Could you check a few things on this model? Use its own coordinates, in mm. A direction names the side the tool comes from. Give positions to 0.01 mm unless a question says otherwise; leave off trailing zeros. Order: outer loops, then holes, each group sorted by start corner. A loop starts at its lowest first (then second) coordinate and runs counter-clockwise, first axis right, second up. Notation, with made-up numbers: (70.25, 25) -> (106.25, 25) arc R15 cw to (106.25, 29) -> close; hole circle Ø9 at (62.5, 23). An arc over 180 degrees is marked (long way). Answer as CSV lines item,"result". Start each with the question number.
(1) I want a section at B-B (y = 202). Please give me the cut outline in (x, z), plus the area to 3 significant figures.
(2) We'd pull the mould along X, two halves only. Please class faces 1 (the face through (-74, 255, 19.5)), 2 (the face through (83.33, 263.645, 6.844)), 3 (the face through (0.2, 0.7, 10.5)), 4 (the face through (-100.776, 165.584, 17.937)): released by +X, released by -X, zero draft, split by the parting line, or undercut.
(3) I want a section at C-C (z = 4.5). Give the number of separate pieces and of enclosed holes in the cut face, plus the area to 3 significant figures.
(4) On a 3-axis mill with a long thin cutter (end or side, diameter ignored), from which of +Z, -Z, +X, -X, +Y, -Y can I reach the whole of each face in a straight line? I mean faces 5 (the face through (42, 43, 9.5)), 6 (the face through (-1, 280.197, 11)), 7 (the face through (44, 13, 10)). Say none if no direction works.
(5) I want a section at A-A (x = -24). Please give me the cut outline in (y, z).
(6) Will these pins go through, and if not, where does the flat tip stop? pin 1 Ø3.5 at (y, z) = (5.5, 5.5) entering from -X; pin 2 Ø8 at (x, z) = (23, 18.5) entering from -Y; pin 3 Ø7 at (y, z) = (40.5, 6) entering from +X.
(7) I need wall thicknesses on L1, parallel to X at y = 53, z = 12.5; L2, parallel to X at y = 194.5, z = 8.25; L3, parallel to Y at x = 45.5, z = 15. Which ranges of each line are inside material? Lowest first, please.
```python
from build123d import *

# Parameters (mm, degrees)
RESSALTO_EXTRUS_O1_DEPTH = 22.5
CHANFRO1_SIZE            = 9
CORTE_EXTRUS_O1_REACH    = 24.5
ESBO_O3_W                = 1139.230904301
ESBO_O3_H                = 709.798033895
CORTE_EXTRUS_O5_DEPTH    = 3
CORTE_EXTRUS_O6_REACH    = 21.5
ESBO_O5_W                = 77
ESBO_O5_H                = 10
ESBO_O7_R                = 2.1
ESBO_O7_R_2              = 2.15
CORTE_EXTRUS_O7_DEPTH    = 23.5
CORTE_EXTRUS_O8_DEPTH    = 10
ESBO_O9_W                = 92.788829696
ESBO_O9_H                = 85.062360753
CORTE_EXTRUS_O9_DEPTH    = 23.5
CORTE_EXTRUS_O10_REACH   = 21.5
CORTE_EXTRUS_O11_DEPTH   = 7
ESBO_O12_R               = 10.5
CORTE_EXTRUS_O12_DEPTH   = 7
CORTE_EXTRUS_O13_DEPTH   = 10


with BuildPart() as part:
    # Esboço1 → Ressalto-extrusão1 (new body, symmetric)
    with BuildSketch(Plane.XY):
        with BuildLine():
            Line((-56.387503511, 290.197344596), (56.387503511, 290.197344596))
            ThreePointArc((56.387503511, 290.197344596), (60.613686129, 289.260422466), (64.047947942, 286.625220692))
            Line((64.047947942, 286.625220692), (103.160444431, 240.012762487))
            ThreePointArc((103.160444431, 240.012762487), (104.896926208, 237.005087823), (105.5, 233.58488639))
            Line((105.5, 233.58488639), (105.5, 167.188670131))
            ThreePointArc((105.5, 167.188670131), (104.953136861, 164.08725515), (103.378507208, 161.359916588))
            Line((103.378507208, 161.359916588), (62.621492792, 112.787598236))
            ThreePointArc((62.621492792, 112.787598236), (61.046863139, 110.060259674), (60.5, 106.958844693))
            Line((60.5, 106.958844693), (60.5, 10.605625498))
            ThreePointArc((60.5, 10.605625498), (59.56307787, 6.379442881), (56.927876097, 2.945181067))
            Line((56.927876097, 2.945181067), (55.249552272, 1.536900164))
            ThreePointArc((55.249552272, 1.536900164), (52.241877608, -0.199581612), (48.821676175, -0.802655404))
            Line((48.821676175, -0.802655404), (-48.821676175, -0.802655404))
            ThreePointArc((-48.821676175, -0.802655404), (-52.241877608, -0.199581612), (-55.249552272, 1.536900164))
            Line((-55.249552272, 1.536900164), (-56.927876097, 2.945181067))
            ThreePointArc((-56.927876097, 2.945181067), (-59.56307787, 6.379442881), (-60.5, 10.605625498))
            Line((-60.5, 10.605625498), (-60.5, 106.958844693))
            ThreePointArc((-60.5, 106.958844693), (-61.046863139, 110.060259674), (-62.621492792, 112.787598236))
            Line((-62.621492792, 112.787598236), (-103.378507208, 161.359916588))
            ThreePointArc((-103.378507208, 161.359916588), (-104.953136861, 164.08725515), (-105.5, 167.188670131))
            Line((-105.5, 167.188670131), (-105.5, 233.58488639))
            ThreePointArc((-105.5, 233.58488639), (-104.896926208, 237.005087823), (-103.160444431, 240.012762487))
            Line((-103.160444431, 240.012762487), (-64.047947942, 286.625220692))
            ThreePointArc((-64.047947942, 286.625220692), (-60.613686129, 289.260422466), (-56.387503511, 290.197344596))
        make_face()
        Polygon((-48.869071975, 270.197344596), (48.869071975, 270.197344596), (83.5, 228.925811707), (83.5, 171.895558399), (38.5, 118.266646732), (38.5, 19.197344596), (-38.5, 19.197344596), (-38.5, 118.266646732), (-83.5, 171.895558399), (-83.5, 228.925811707), align=None, mode=Mode.SUBTRACT)
    extrude(amount=RESSALTO_EXTRUS_O1_DEPTH, both=True)

    # Chanfro1
    chanfro1_edges = [part.edges().sort_by_distance(p)[0] for p in [
        (83.604196187, 263.318991589, 22.5),
        (60.613686129, 289.260422466, 22.5),
        (0, 290.197344596, 22.5),
        (-60.613686129, 289.260422466, 22.5),
        (-83.604196187, 263.318991589, 22.5),
        (-104.896926208, 237.005087823, 22.5),
        (-105.5, 200.38677826, 22.5),
        (-104.953136861, 164.08725515, 22.5),
        (-83, 137.073757412, 22.5),
        (-61.046863139, 110.060259674, 22.5),
        (-60.5, 58.782235095, 22.5),
        (-59.56307787, 6.379442881, 22.5),
        (-56.088714184, 2.241040616, 22.5),
        (-52.241877608, -0.199581612, 22.5),
        (0, -0.802655404, 22.5),
        (52.241877608, -0.199581612, 22.5),
        (56.088714184, 2.241040616, 22.5),
        (59.56307787, 6.379442881, 22.5),
        (60.5, 58.782235095, 22.5),
        (61.046863139, 110.060259674, 22.5),
        (83, 137.073757412, 22.5),
        (104.953136861, 164.08725515, 22.5),
        (105.5, 200.38677826, 22.5),
        (104.896926208, 237.005087823, 22.5),
    ]]
    chamfer(chanfro1_edges, length=CHANFRO1_SIZE)

    # Esboço3 → Corte-extrusão1 (cut, up to next)
    with BuildSketch(Plane.XY, mode=Mode.PRIVATE) as corte_extrus_o1_sk1:
        with Locations((-153.157436203, 152.53565808)):
            Rectangle(ESBO_O3_W, ESBO_O3_H)
    corte_extrus_o1_tool1 = extrude(corte_extrus_o1_sk1.sketch, amount=-CORTE_EXTRUS_O1_REACH, mode=Mode.PRIVATE) & part.part
    add(corte_extrus_o1_tool1.solids().sort_by_distance((-153.157436, 152.535658, 0))[0], mode=Mode.SUBTRACT)

    # Esboço4 → Corte-extrusão5 (cut)
    with BuildSketch(Plane.XY.offset(22.5)):
        Polygon((56.387503511, 280.197344596), (-56.387503511, 280.197344596), (-95.5, 233.58488639), (-95.5, 167.527915588), (-50.5, 113.899003921), (-50.5, 10.605625498), (-48.821676175, 9.197344596), (48.821676175, 9.197344596), (50.5, 10.605625498), (50.5, 113.899003921), (95.5, 167.527915588), (95.5, 233.58488639), align=None)
        Polygon((38.5, 19.197344596), (-38.5, 19.197344596), (-38.5, 121.489121124), (-83.5, 175.11803279), (-83.5, 228.925811707), (-48.869071975, 270.197344596), (48.869071975, 270.197344596), (83.5, 228.925811707), (83.5, 175.11803279), (38.5, 121.489121124), align=None, mode=Mode.SUBTRACT)
    extrude(amount=-CORTE_EXTRUS_O5_DEPTH, mode=Mode.SUBTRACT)

    # Esboço5 → Corte-extrusão6 (cut, up to next)
    with BuildSketch(Plane.XY.offset(19.5), mode=Mode.PRIVATE) as corte_extrus_o6_sk1:
        Polygon((-95.5, 233.58488639), (-83.5, 228.925811707), (-83.5, 171.895558399), (-95.5, 167.527915588), align=None)
    corte_extrus_o6_tool1 = extrude(corte_extrus_o6_sk1.sketch, amount=-CORTE_EXTRUS_O6_REACH, mode=Mode.PRIVATE) & part.part
    add(corte_extrus_o6_tool1.solids().sort_by_distance((-89.646672, 200.485324, 19.5))[0], mode=Mode.SUBTRACT)
    # Esboço5 → Corte-extrusão6 (cut, up to next)
    with BuildSketch(Plane.XY.offset(19.5), mode=Mode.PRIVATE) as corte_extrus_o6_sk2:
        Polygon((-48.869071975, 270.197344596), (-56.387503511, 280.197344596), (56.387503511, 280.197344596), (48.869071975, 270.197344596), align=None)
    corte_extrus_o6_tool2 = extrude(corte_extrus_o6_sk2.sketch, amount=-CORTE_EXTRUS_O6_REACH, mode=Mode.PRIVATE) & part.part
    add(corte_extrus_o6_tool2.solids().sort_by_distance((0, 275.316394, 19.5))[0], mode=Mode.SUBTRACT)
    # Esboço5 → Corte-extrusão6 (cut, up to next)
    with BuildSketch(Plane.XY.offset(19.5), mode=Mode.PRIVATE) as corte_extrus_o6_sk3:
        with Locations((0, 14.197344596)):
            Rectangle(ESBO_O5_W, ESBO_O5_H)
    corte_extrus_o6_tool3 = extrude(corte_extrus_o6_sk3.sketch, amount=-CORTE_EXTRUS_O6_REACH, mode=Mode.PRIVATE) & part.part
    add(corte_extrus_o6_tool3.solids().sort_by_distance((0, 14.197345, 19.5))[0], mode=Mode.SUBTRACT)
    # Esboço5 → Corte-extrusão6 (cut, up to next)
    with BuildSketch(Plane.XY.offset(19.5), mode=Mode.PRIVATE) as corte_extrus_o6_sk4:
        Polygon((83.5, 171.895558399), (95.5, 167.527915588), (95.5, 233.58488639), (83.5, 228.925811707), align=None)
    corte_extrus_o6_tool4 = extrude(corte_extrus_o6_sk4.sketch, amount=-CORTE_EXTRUS_O6_REACH, mode=Mode.PRIVATE) & part.part
    add(corte_extrus_o6_tool4.solids().sort_by_distance((89.646672, 200.485324, 19.5))[0], mode=Mode.SUBTRACT)

    # Esboço7 → Corte-extrusão7 (cut, through all)
    with BuildSketch(Plane.XY.offset(22.5)):
        with Locations((-45.5, 14.923339275)):
            Circle(ESBO_O7_R)
        with Locations((-43.5, 44.856598369)):
            Circle(ESBO_O7_R_2)
        with Locations((-71.975269931, 253.84194883)):
            Circle(ESBO_O7_R)
        with Locations((-59.836146954, 265.197344596)):
            Circle(ESBO_O7_R_2)
        with Locations((59.836146954, 265.197344596)):
            Circle(ESBO_O7_R_2)
        with Locations((71.975269931, 253.84194883)):
            Circle(ESBO_O7_R)
        with Locations((43.5, 44.856598369)):
            Circle(ESBO_O7_R_2)
        with Locations((45.5, 14.923339275)):
            Circle(ESBO_O7_R)
        with Locations((-67.431100943, 144.966771084)):
            Circle(ESBO_O7_R_2)
        with Locations((67.431100943, 144.966771084)):
            Circle(ESBO_O7_R_2)
    extrude(amount=-CORTE_EXTRUS_O7_DEPTH, mode=Mode.SUBTRACT)

    # Esboço8 → Corte-extrusão8 (cut)
    with BuildSketch(Plane(origin=(0, 0, 0), x_dir=(-1, 0, 0), z_dir=(0, 0, -1))):
        Polygon((-73.397020968, 257.748177701), (-76.069038884, 254.56379075), (-74.647287847, 250.657561879), (-70.553518893, 249.93571996), (-67.881500977, 253.120106911), (-69.303252014, 257.026335782), align=None)
        Polygon((-45.5, 19.080261213), (-49.1, 17.001800244), (-49.1, 12.844878306), (-45.5, 10.766417337), (-41.9, 12.844878306), (-41.9, 17.001800244), align=None)
        Polygon((41.9, 17.001800244), (45.5, 19.080261213), (49.1, 17.001800244), (49.1, 12.844878306), (45.5, 10.766417337), (41.9, 12.844878306), align=None)
        Polygon((76.069038884, 254.56379075), (73.397020968, 257.748177701), (69.303252014, 257.026335782), (67.881500977, 253.120106911), (70.553518893, 249.93571996), (74.647287847, 250.657561879), align=None)
        Polygon((67.580931876, 147.478918378), (71.560985025, 146.777127623), (72.943242978, 142.97940511), (70.345447782, 139.883473352), (66.365394632, 140.585264107), (64.98313668, 144.38298662), align=None)
    extrude(amount=-CORTE_EXTRUS_O8_DEPTH, mode=Mode.SUBTRACT)

    # Esboço9 → Corte-extrusão9 (cut, through all)
    with BuildSketch(Plane.XY.offset(22.5)):
        with Locations((-70.062226852, 117.896927121)):
            Rectangle(ESBO_O9_W, ESBO_O9_H)
    extrude(amount=-CORTE_EXTRUS_O9_DEPTH, mode=Mode.SUBTRACT)

    # Esboço10 → Corte-extrusão10 (cut, up to next)
    with BuildSketch(Plane.XY.offset(19.5), mode=Mode.PRIVATE) as corte_extrus_o10_sk1:
        Polygon((-95.5, 167.527915588), (-83.5, 171.895558399), (-73.877666178, 160.428107498), (-89.54255365, 160.428107498), align=None)
    corte_extrus_o10_tool1 = extrude(corte_extrus_o10_sk1.sketch, amount=-CORTE_EXTRUS_O10_REACH, mode=Mode.PRIVATE) & part.part
    add(corte_extrus_o10_tool1.solids().sort_by_distance((-85.062746, 165.15554, 19.5))[0], mode=Mode.SUBTRACT)
    # Esboço10 → Corte-extrusão10 (cut, up to next)
    with BuildSketch(Plane.XY.offset(19.5), mode=Mode.PRIVATE) as corte_extrus_o10_sk2:
        Polygon((89.54255365, 160.428107498), (95.5, 167.527915588), (83.5, 171.895558399), (73.877666178, 160.428107498), align=None)
    corte_extrus_o10_tool2 = extrude(corte_extrus_o10_sk2.sketch, amount=-CORTE_EXTRUS_O10_REACH, mode=Mode.PRIVATE) & part.part
    add(corte_extrus_o10_tool2.solids().sort_by_distance((85.062746, 165.15554, 19.5))[0], mode=Mode.SUBTRACT)

    # Esboço11 → Corte-extrusão11 (cut)
    with BuildSketch(Plane(origin=(0, 9.197344596, 0), x_dir=(1, 0, 0), z_dir=(0, 1, 0))):
        Polygon((0, -15.703927322), (13.6, -7.851963661), (13.6, 7.851963661), (0, 15.703927322), (-13.6, 7.851963661), (-13.6, -7.851963661), align=None)
    extrude(amount=-CORTE_EXTRUS_O11_DEPTH, mode=Mode.SUBTRACT)

    # Esboço12 → Corte-extrusão12 (cut)
    with BuildSketch(Plane.XZ.offset(0.802655404)):
        Circle(ESBO_O12_R)
    extrude(amount=-CORTE_EXTRUS_O12_DEPTH, mode=Mode.SUBTRACT)

    # Esboço13 → Corte-extrusão13 (cut)
    with BuildSketch(Plane.XY.offset(19.5)):
        Polygon((-57.089906317, 268.47018674), (-61.297391075, 269.212079824), (-64.043631711, 265.939237679), (-62.58238759, 261.924502451), (-58.374902832, 261.182609368), (-55.628662196, 264.455451512), align=None)
        Polygon((61.297391075, 269.212079824), (57.089906317, 268.47018674), (55.628662196, 264.455451512), (58.374902832, 261.182609368), (62.58238759, 261.924502451), (64.043631711, 265.939237679), align=None)
        Polygon((-47.2, 46.992794365), (-47.2, 42.720402373), (-43.5, 40.584206377), (-39.8, 42.720402373), (-39.8, 46.992794365), (-43.5, 49.128990361), align=None)
        Polygon((47.2, 46.992794365), (43.5, 49.128990361), (39.8, 46.992794365), (39.8, 42.720402373), (43.5, 40.584206377), (47.2, 42.720402373), align=None)
        Polygon((70.177341579, 148.239613229), (65.969856821, 148.981506312), (63.223616185, 145.708664168), (64.684860306, 141.69392894), (68.892345064, 140.952035856), (71.6385857, 144.224878001), align=None)
    extrude(amount=-CORTE_EXTRUS_O13_DEPTH, mode=Mode.SUBTRACT)


solid = part.part
```
Final values:
1,outline,"(-105.5, 0) -> (-95.5, 0) -> (-95.5, 22.5) -> (-96.5, 22.5) -> (-105.5, 13.5) -> close; (95.5, 0) -> (105.5, 0) -> (105.5, 13.5) -> (96.5, 22.5) -> (95.5, 22.5) -> close"
1,area,"369 mm²"
2,face 1,"undercut"
2,face 2,"released by +X"
2,face 3,"undercut"
2,face 4,"released by -X"
3,separate pieces,"2"
3,enclosed holes,"9"
3,area,"11,100 mm²"
4,face 5,"+Z"
4,face 6,"+Z, -Z"
4,face 7,"-Z"
5,outline,"(-0.8, 0) -> (9.2, 0) -> (9.2, 22.5) -> (8.2, 22.5) -> (-0.8, 13.5) -> close; (280.2, 0) -> (290.2, 0) -> (290.2, 13.5) -> (281.2, 22.5) -> (280.2, 22.5) -> close"
6,pin 1,"x = -59.92"
6,pin 2,"y = 0.2"
6,pin 3,"x = 60.5"
7,L1,"-60.5 to -38.5, 38.5 to 60.5"
7,L2,"-105.5 to -95.5, 95.5 to 105.5"
7,L3,"0.7 to 12.82, 17.02 to 41.74, 47.97 to 126.61, 280.2 to 288.7"
